Build history of the part. All positions in model axes, mm. A direction names the side the tool comes from. Give positions to 0.01 mm unless a question says otherwise; leave off trailing zeros. Write each loop counter-clockwise with the first axis right and the second up, starting at its lowest first coordinate (ties: lowest second). Pieces come first, ordered by that corner, then holes.
from build123d import *

# Parameters (mm, degrees)
F0_W     = 41
F0_H     = 16
F1_DEPTH = 4
F2_D     = 3.5
F2_DEPTH = 3.5
F2_TIP   = 1.0515060833
F3_SIZE  = 6


with BuildPart() as f1:
    # F0 (on Top) → F1 (new body)
    with BuildSketch(Plane.XY):
        Rectangle(F0_W, F0_H)
    extrude(amount=F1_DEPTH)

    # F2
    with Locations(Plane(origin=(0, 0, 0), x_dir=(1, 0, 0), z_dir=(0, 0, -1))):
        with Locations((-10.5, 2), (9.5, 2)):
            Hole(F2_D / 2, depth=F2_DEPTH)
            with Locations((0, 0, -(F2_DEPTH + F2_TIP / 2))):  # 118° drill point
                Cone(0, F2_D / 2, F2_TIP, mode=Mode.SUBTRACT)

    # F3
    f3_edges = [f1.edges().sort_by_distance(p)[0] for p in [
        (20.5, 8, 2),
    ]]
    chamfer(f3_edges, length=F3_SIZE)


solid = f1.part
(1) Saw through at B-B, the plane y = -2. List the corners of the cut face in (x, z), plus the area to 3 significant figures.
(2) Mould opens along Y. For faces 1 (the face through (20.5, -3, 2)), 2 (the face through (17.5, 5, 2)), 3 (the face through (7.883, -1.33, 1.774)) say: +Y half, -Y half, draft (parallel to the pull), parting line (faces both ways), or undercut.
(3) 3-axis set-ups, long thin cutter, end or side, ignore diameter. For faces 4 (the face through (-3, 8, 2)), 5 (the face through (-12.117, -1.33, 1.774)): which of +Z, -Z, +X, -X, +Y, -Y reach the whole face in a straight line?
(4) Saw through at C-C, the plane x = -10.5. List the corners of the cut face in (y, z), plus the area to 3 significant figures.
(5) Saw through at D-D, the plane y = 5. List the corners of the cut face in (x, z).
(6) Probe line 1 (Y direction, x = -10.5, z = 2.2); line 2 (X direction, y = -1, z = 1.85); line 3 (Y direction, x = 11, z = 1.2). List the from-to ranges inside material, lowest first.
(7) Saw through at A-A, the plane z = 1.65. List the corners of the cut face in (x, y), plus the area to 3 significant figures.
Computed values:
1. outline: (-20.5, 0) - (-12.25, 0) - (-12.25, 3.5) - (-11.42, 4) - (-20.5, 4) - close; (-9.58, 4) - (-8.75, 3.5) - (-8.75, 0) - (7.75, 0) - (7.75, 3.5) - (8.58, 4) - close; (10.42, 4) - (11.25, 3.5) - (11.25, 0) - (20.5, 0) - (20.5, 4) - close
1. area: 137 mm2
2. face 1: draft
2. face 2: +Y half
2. face 3: undercut
3. face 4: +Z, -Z, +X, -X, +Y
3. face 5: -Z
4. outline: (-8, 0) - (-3.75, 0) - (-3.75, 3.5) - (-2.92, 4) - (-8, 4) - close; (-1.08, 4) - (-0.25, 3.5) - (-0.25, 0) - (8, 0) - (8, 4) - close
4. area: 50.4 mm2
5. outline: (-20.5, 0) - (17.5, 0) - (17.5, 4) - (-20.5, 4) - close
6. line 1: y = -8 to -3.75, -0.25 to 8
6. line 2: x = -20.5 to -11.94, -9.06 to 8.06, 10.94 to 20.5
6. line 3: y = -8 to -2.9, -1.1 to 8
7. outline: (-20.5, -8) - (20.5, -8) - (20.5, 2) - (14.5, 8) - (-20.5, 8) - close; hole circle Ø3.5 at (-10.5, -2); hole circle Ø3.5 at (9.5, -2)
7. area: 619 mm2
